```python
from build123d import *

# Parameters (mm, degrees)
EXTRUDE_1_DEPTH = 20
EXTRUDE_START   = -2
SKETCH_1_3_R    = 16
SKETCH_1_3_R_2  = 21
EXTRUDE_2_DEPTH = 2
SWEEP_1_ANGLE   = 286.260205
EXTRUDE_4_DEPTH = 5
EXTRUDE_5_DEPTH = 5


# Read off the part's stored shape, not the designer's step: По траектории1
with BuildPart() as part:
    # Эскиз1 → Бобышка-Вытянуть1 (new body)
    with BuildSketch(Plane(origin=(0, 0, 0), x_dir=(1, 0, 0), z_dir=(0, 1, 0))):
        with BuildLine():
            ThreePointArc((-15.332019477, -0.360375994), (-30.332019477, 14.639624006), (-15.332019477, 29.639624006))
            Line((-15.332019477, 29.639624006), (-15.332019477, 30.639624006))
            ThreePointArc((-15.332019477, 30.639624006), (-31.332019477, 14.639624006), (-15.332019477, -1.360375994))
            Line((-15.332019477, -1.360375994), (-15.332019477, -0.360375994))
        make_face()
        with BuildLine():
            Line((-15.332019477, 30.639624006), (-15.332019477, 29.639624006))
            ThreePointArc((-15.332019477, 29.639624006), (-11.459036131, 29.131000752), (-7.848704703, 27.639624006))
            Line((-7.848704703, 27.639624006), (-6.824441979, 27.639624006))
            ThreePointArc((-6.824441979, 27.639624006), (-6.679236311, 27.821752127), (-6.532019477, 28.002258477))
            ThreePointArc((-6.532019477, 28.002258477), (-10.738662944, 29.96610683), (-15.332019477, 30.639624006))
        make_face()
        with BuildLine():
            ThreePointArc((-7.848704703, 1.639624006), (-11.459036131, 0.14824726), (-15.332019477, -0.360375994))
            Line((-15.332019477, -0.360375994), (-15.332019477, -1.360375994))
            ThreePointArc((-15.332019477, -1.360375994), (-10.738662944, -0.686858818), (-6.532019477, 1.276989535))
            ThreePointArc((-6.532019477, 1.276989535), (-6.679236311, 1.457495885), (-6.824441979, 1.639624006))
            Line((-6.824441979, 1.639624006), (-7.848704703, 1.639624006))
        make_face()
        with BuildLine():
            ThreePointArc((-6.004640424, 1.639624006), (-6.266516525, 1.455669507), (-6.532019477, 1.276989535))
            ThreePointArc((-6.532019477, 1.276989535), (0.712963044, -4.355313792), (9.667980523, -6.360375994))
            Line((9.667980523, -6.360375994), (9.667980523, -5.360375994))
            ThreePointArc((9.667980523, -5.360375994), (1.301380258, -3.526278119), (-5.53070363, 1.639624006))
            Line((-5.53070363, 1.639624006), (-6.004640424, 1.639624006))
        make_face()
        with BuildLine():
            ThreePointArc((30.667980523, 14.639624006), (16.767276263, 34.403226916), (-6.532019477, 28.002258477))
            ThreePointArc((-6.532019477, 28.002258477), (-6.266516525, 27.823578505), (-6.004640424, 27.639624006))
            Line((-6.004640424, 27.639624006), (-5.53070363, 27.639624006))
            ThreePointArc((-5.53070363, 27.639624006), (16.597133319, 33.400936368), (29.667980523, 14.639624006))
            ThreePointArc((29.667980523, 14.639624006), (23.810116147, 0.497488382), (9.667980523, -5.360375994))
            Line((9.667980523, -5.360375994), (9.667980523, -6.360375994))
            ThreePointArc((9.667980523, -6.360375994), (24.517222928, -0.209618399), (30.667980523, 14.639624006))
        make_face()
        with BuildLine():
            ThreePointArc((-6.532019477, 28.002258477), (-6.679236311, 27.821752127), (-6.824441979, 27.639624006))
            Line((-6.824441979, 27.639624006), (-6.004640424, 27.639624006))
            ThreePointArc((-6.004640424, 27.639624006), (-6.266516525, 27.823578505), (-6.532019477, 28.002258477))
        make_face()
        with BuildLine():
            Line((-6.824441979, 27.639624006), (-7.848704703, 27.639624006))
            ThreePointArc((-7.848704703, 27.639624006), (-7.497456441, 27.431012595), (-7.152019477, 27.212913154))
            ThreePointArc((-7.152019477, 27.212913154), (-6.989597145, 27.427317552), (-6.824441979, 27.639624006))
        make_face()
        with BuildLine():
            ThreePointArc((-6.824441979, 27.639624006), (-6.989597145, 27.427317552), (-7.152019477, 27.212913154))
            ThreePointArc((-7.152019477, 27.212913154), (-6.737238205, 26.933107438), (-6.332019477, 26.639624006))
            ThreePointArc((-6.332019477, 26.639624006), (-6.02692778, 27.035988527), (-5.712019477, 27.424599563))
            ThreePointArc((-5.712019477, 27.424599563), (-5.857719918, 27.532941961), (-6.004640424, 27.639624006))
            Line((-6.004640424, 27.639624006), (-6.824441979, 27.639624006))
        make_face()
        with BuildLine():
            Line((-5.53070363, 27.639624006), (-6.004640424, 27.639624006))
            ThreePointArc((-6.004640424, 27.639624006), (-5.857719918, 27.532941961), (-5.712019477, 27.424599563))
            ThreePointArc((-5.712019477, 27.424599563), (-5.621739553, 27.532430527), (-5.53070363, 27.639624006))
        make_face()
        with BuildLine():
            ThreePointArc((-6.332019477, 2.639624006), (-6.737238205, 2.346140574), (-7.152019477, 2.066334858))
            ThreePointArc((-7.152019477, 2.066334858), (-6.989597145, 1.85193046), (-6.824441979, 1.639624006))
            Line((-6.824441979, 1.639624006), (-6.004640424, 1.639624006))
            ThreePointArc((-6.004640424, 1.639624006), (-5.857719918, 1.746306051), (-5.712019477, 1.854648449))
            ThreePointArc((-5.712019477, 1.854648449), (-6.02692778, 2.243259485), (-6.332019477, 2.639624006))
        make_face()
        with BuildLine():
            ThreePointArc((-7.152019477, 2.066334858), (-7.497456441, 1.848235417), (-7.848704703, 1.639624006))
            Line((-7.848704703, 1.639624006), (-6.824441979, 1.639624006))
            ThreePointArc((-6.824441979, 1.639624006), (-6.989597145, 1.85193046), (-7.152019477, 2.066334858))
        make_face()
        with BuildLine():
            Line((-6.004640424, 1.639624006), (-6.824441979, 1.639624006))
            ThreePointArc((-6.824441979, 1.639624006), (-6.679236311, 1.457495885), (-6.532019477, 1.276989535))
            ThreePointArc((-6.532019477, 1.276989535), (-6.266516525, 1.455669507), (-6.004640424, 1.639624006))
        make_face()
        with BuildLine():
            ThreePointArc((-5.712019477, 1.854648449), (-5.857719918, 1.746306051), (-6.004640424, 1.639624006))
            Line((-6.004640424, 1.639624006), (-5.53070363, 1.639624006))
            ThreePointArc((-5.53070363, 1.639624006), (-5.621739553, 1.746817485), (-5.712019477, 1.854648449))
        make_face()
    extrude(amount=EXTRUDE_1_DEPTH)

    # Эскиз1<3> → Бобышка-Вытянуть2 (add)
    with BuildSketch(Plane(origin=(0, 0, 0), x_dir=(1, 0, 0), z_dir=(0, 1, 0)).offset(EXTRUDE_START)):
        with Locations((-15.332019477, 14.639624006)):
            Circle(SKETCH_1_3_R)
        with Locations((9.667980523, 14.639624006)):
            Circle(SKETCH_1_3_R_2)
    extrude(amount=EXTRUDE_2_DEPTH)

    # По траектории1 outline → По траектории1 (revolve)
    with BuildSketch(Plane(origin=(9.667980523, 0, -14.639624006), x_dir=(-0.7999999999999995, 0, 0.6000000000000008), z_dir=(-0.6000000000000008, 0, -0.7999999999999995))):
        with BuildLine():
            ThreePointArc((20, 5), (16.464466094, 3.535533906), (15, 0))
            Line((15, 0), (20, 0))
            Line((20, 0), (20, 5))
        make_face()
    revolve(axis=Axis((9.667980523, 0, -14.639624006), (0, 1, 0)), revolution_arc=SWEEP_1_ANGLE)

    # По траектории9: sweep along a curve in space
    with BuildLine() as sweep_9_path:
        ThreePointArc((-6.332019477, 0, -26.639624006), (-30.332019477, 0, -14.639624006), (-6.332019477, 0, -2.639624006))
    # Sketch 5 → По траектории9 (sweep)
    with BuildSketch(Plane(origin=(-30.332019477, 0, -14.639624006), x_dir=(1, 0, 0), z_dir=(0, 0, 1))):
        with BuildLine():
            Line((0, 0), (5, 0))
            ThreePointArc((5, 0), (3.535533906, 3.535533906), (0, 5))
            Line((0, 5), (0, 0))
        make_face()
    sweep(path=sweep_9_path.line)

    # Эскиз17 → Бобышка-Вытянуть4 (add)
    with BuildSketch(Plane(origin=(0, 0, 0), x_dir=(1, 0, 0), z_dir=(0, 1, 0))):
        Polygon((-9.332019477, 6.639624006), (-2.332019477, 5.639624006), (-6.332019477, 2.639624006), align=None)
    extrude(amount=EXTRUDE_4_DEPTH)

    # Эскиз19 → Бобышка-Вытянуть5 (add)
    with BuildSketch(Plane(origin=(0, 0, 0), x_dir=(1, 0, 0), z_dir=(0, 1, 0))):
        Polygon((-2.332019477, 23.639624006), (-9.332019477, 22.639624006), (-6.332019477, 26.639624006), align=None)
    extrude(amount=EXTRUDE_5_DEPTH)


solid = part.part
```
Geometry check sheet. Reference: the model listing, model coordinates, mm. A direction names the side the tool comes from. Coordinates: 2 decimals unless noted, no trailing zeros. Write each loop counter-clockwise with the first axis right and the second up, starting at its lowest first coordinate (ties: lowest second). Pieces come first, ordered by that corner, then holes. Notation, with made-up numbers: M -39,53.5 L -1,53.5 A23 ccw -1,80.5 Z; hole C 55.5,74 d6. An arc over 180 degrees is marked long. Answer as a JSON object with one key per item and string values.
1. Draft check along Z on faces 3 (the flat face through (-3.16, 3.97, -24.26)), 4 (the flat face through (-6, 5, -24)), 5 (the flat face through (-5.1, 20, -0.7)). Enter one of: released by +Z, released by -Z, zero draft, split by the parting line, or undercut.
Answers below:
{"face 3": "undercut", "face 4": "undercut", "face 5": "zero draft"}
2. Tool access check on faces 1 (the flat face through (-8.7, 4, -5.8)), 2 (the flat face through (-1, -2, -15)). Record the directions out of +Z, -Z, +X, -X, +Y, -Y that give a thin tool (end or side, any length) a straight path to the whole face; none if there is none.
Answers below:
{"face 1": "+Y", "face 2": "+Z, -Z, +X, -X, -Y"}
3. Scan lines: L1, parallel to Z at x = -15, y = 10; L2, parallel to Z at x = -10.5, y = 15; L3, parallel to X at y = 8.75, z = -2.5. Record each from-to range of solid material in increasing order.
Answers below:
{"L1": "z = -30.64 to -29.64, 0.36 to 1.36", "L2": "z = -29.89 to -28.84, -0.44 to 0.61", "L3": "x = -25.75 to -24.14, -6.52 to -6.23, 25.56 to 26.8"}
4. Section check A-A, the plane y = 9.5. Enter the section's corners in (x, z).
Answers below:
{"outline": "M -6.53,-28 A21 ccw long -6.53,-1.28 A16 ccw long Z; hole M -6.33,-26.64 A20 ccw -5.71,-27.42 A20 ccw -5.53,-27.64 A20 ccw long -5.53,-1.64 A20 ccw -5.71,-1.85 A20 ccw -6.33,-2.64 A15 ccw long Z"}
5. Go/stop test with flat-tipped pins: pin 1 Ø9 at (x, z) = (10.5, -17) entering from +Y; pin 2 Ø10 at (x, y) = (24.5, 3.5) entering from -Z; pin 3 Ø5 at (y, z) = (1.5, -26.5) entering from -X. Record where each tip stops, or that it passes through.
Answers below:
{"pin 1": "stops at y = 0", "pin 2": "stops at z = -33.2", "pin 3": "stops at x = -28.31"}
